Can you work these out from the model? Positions are in its coordinate system, mm. Face numbers are marked on the shaded views. A direction names the side the tool comes from. Give positions to 0.01 mm unless a question says otherwise; leave off trailing zeros. Write each loop counter-clockwise with the first axis right and the second up, starting at its lowest first coordinate (ties: lowest second). Pieces come first, ordered by that corner, then holes.
1. Suppose I cut it at D-D (z = 5.5). Please give me the cut outline in (x, y) (3 decimals), and give its area (3 significant figures).
2. I'm going to push flat-ended pins straight in: pin 1 (2 mm diameter, centred on x = 19.5, z = 7, fed in from +Y) (3 decimals); pin 2 (1.5 mm diameter, centred on x = 4, y = 21.5, fed in from -Z); pin 3 (10 mm diameter, centred on x = 25.5, y = 5, fed in from +Z); pin 4 (12.5 mm diameter, centred on y = 22, z = 7, fed in from +X) (3 decimals). Where does each tip first touch, or does it pass through?
3. Suppose I cut it at B-B (y = 25.4). Please give me the cut outline in (x, z) (3 decimals), and give its area (3 significant figures).
4. Suppose I cut it at A-A (z = 19.05). Please give me the cut outline in (x, y) (1 decimal).
5. If I drill on probe 1 along Z at (x, y) = (27, 3); probe 2 along X at (y, z) = (1.7, 12.7); probe 3 along Y at (x, z) = (0.9, 12.7) (3 decimals), over which ranges is the centre line in solid material (lowest first)?
6. Suppose I cut it at C-C (z = 14.5). Please give me the cut outline in (x, y) (3 decimals).
7. On a 3-axis mill with a long thin cutter (end or side, diameter ignored), from which of +Z, -Z, +X, -X, +Y, -Y can I reach the whole of each face in a straight line? I mean the marked faces 1 and 2. Say none if no direction works.
```python
from build123d import *

# Parameters (mm, degrees)
EXTRUDE_THIN1_DEPTH = 25.4
SKETCH2_R           = 4.7625
CUT_EXTRUDE1_DEPTH  = 4.175
SKETCH3_R           = 2.4765
CUT_EXTRUDE2_DEPTH  = 39.1
SKETCH4_R           = 3.175
CUT_EXTRUDE3_DEPTH  = 39.1


with BuildPart() as part:
    # Sketch1 → Extrude-Thin1 (new body)
    with BuildSketch(Plane.XY):
        Polygon((0, 38.1), (0, 0), (38.1, 0), (38.1, 3.175), (3.175, 3.175), (3.175, 38.1), align=None)
    extrude(amount=EXTRUDE_THIN1_DEPTH)

    # Sketch2 → Cut-Extrude1 (cut, through all)
    with BuildSketch(Plane(origin=(0, 3.175, 0), x_dir=(1, 0, 0), z_dir=(0, 1, 0))):
        with Locations((9.525, -12.7)):
            Circle(SKETCH2_R)
    extrude(amount=-CUT_EXTRUDE1_DEPTH, mode=Mode.SUBTRACT)

    # Sketch3 → Cut-Extrude2 (cut, through all)
    with BuildSketch(Plane.XZ):
        with Locations((28.575, 19.05)):
            Circle(SKETCH3_R)
        with Locations((28.575, 6.35)):
            Circle(SKETCH3_R)
    extrude(amount=-CUT_EXTRUDE2_DEPTH, mode=Mode.SUBTRACT)

    # Sketch4 → Cut-Extrude3 (cut, through all)
    with BuildSketch(Plane.ZY):
        with Locations((12.7, 25.4)):
            Circle(SKETCH4_R)
    extrude(amount=-CUT_EXTRUDE3_DEPTH, mode=Mode.SUBTRACT)


solid = part.part
```
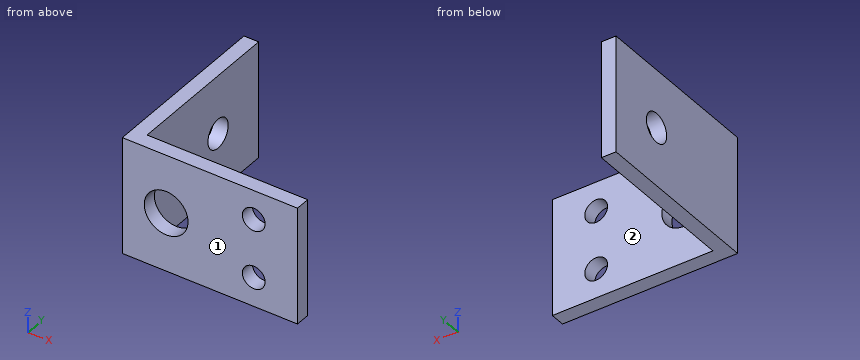
Checks:
1. outline: (0, 0) - (26.249, 0) - (26.249, 3.175) - (3.175, 3.175) - (3.175, 38.1) - (0, 38.1) - close; (30.901, 0) - (38.1, 0) - (38.1, 3.175) - (30.901, 3.175) - close
1. area: 217 mm2
2. pin 1: stops at y = 3.175
2. pin 2: passes through
2. pin 3: stops at z = 25.4
2. pin 4: stops at x = 3.175
3. outline: (0, 0) - (3.175, 0) - (3.175, 9.525) - (0, 9.525) - close; (0, 15.875) - (3.175, 15.875) - (3.175, 25.4) - (0, 25.4) - close
3. area: 60.5 mm2
4. outline: (0, 0) - (26.1, 0) - (26.1, 3.2) - (3.2, 3.2) - (3.2, 38.1) - (0, 38.1) - close; (31.1, 0) - (38.1, 0) - (38.1, 3.2) - (31.1, 3.2) - close
5. probe 1: z = 0 to 4.44, 8.26 to 17.14, 20.96 to 25.4
5. probe 2: x = 0 to 4.76, 14.29 to 38.1
5. probe 3: y = 0 to 22.225, 28.575 to 38.1
6. outline: (0, 0) - (5.116, 0) - (5.116, 3.175) - (3.175, 3.175) - (3.175, 22.785) - (0, 22.785) - close; (0, 28.015) - (3.175, 28.015) - (3.175, 38.1) - (0, 38.1) - close; (13.934, 0) - (38.1, 0) - (38.1, 3.175) - (13.934, 3.175) - close
7. face 1: +Z, -Z, +X, -X, -Y
7. face 2: +Z, -Z, +X, +Y
